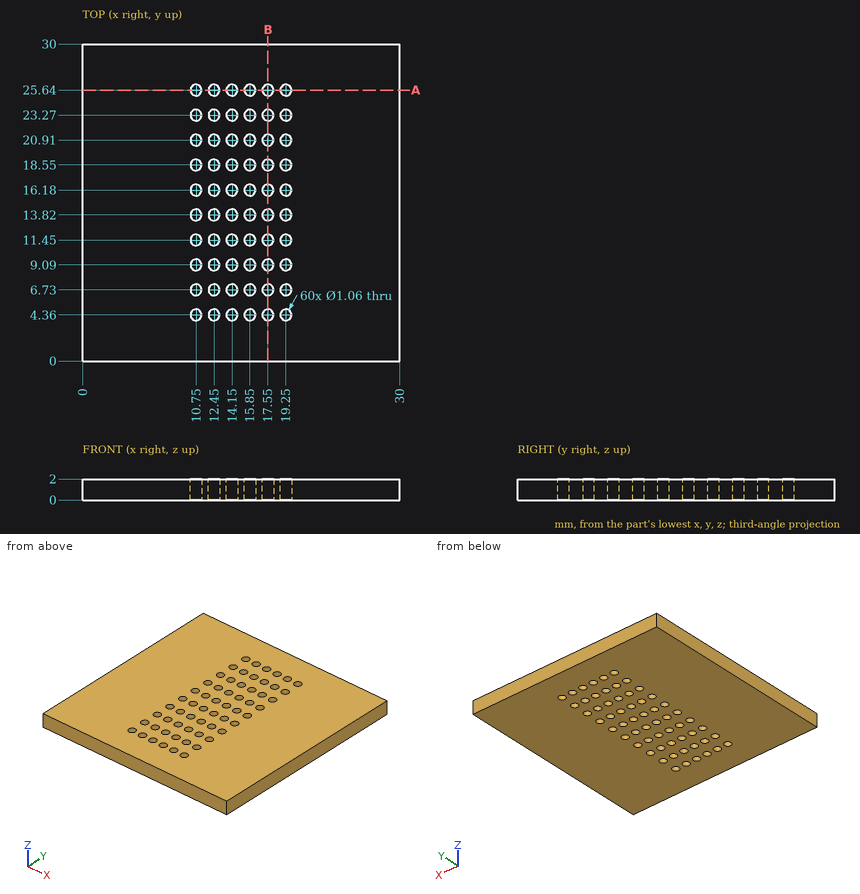
The drawing under review shows one solid part. Ordinate dimensions are in mm from its lowest x, y, z. Round coordinates to 2 decimals unless told otherwise and drop trailing zeros. Write each loop counter-clockwise with the first axis right and the second up, starting at its lowest first coordinate (ties: lowest second). Pieces come first, ordered by that corner, then holes. Notation, with made-up numbers: (1, 35) -> (22, 35) arc R8 cw to (22, 49) -> close; hole circle Ø9 at (31.5, 65.25). An arc over 180 degrees is marked (long way). One line per question, with ' | ' between items.
(1) Insertion check: P1, Ø1.2, axis at x = 12.45, y = 23.27, coming from the +Z side. The pin has a flat end and moves straight along its axis. Give the tip position at first contact, or say it passes through.
Result sheet:
P1: z = 2
(2) Take a section at B-B, the plane x = 17.55. State how many separate pieces and enclosed holes the cut face has, and give its area (3 significant figures).
Result sheet:
separate pieces: 11 | enclosed holes: 0 | area: 38.8 mm2
(3) Take a section at A-A, the plane y = 25.64. State the section outline as (x, z) points, and give its area (3 significant figures).
Result sheet:
outline: (0, 0) -> (10.22, 0) -> (10.22, 2) -> (0, 2) -> close; (11.28, 0) -> (11.92, 0) -> (11.92, 2) -> (11.28, 2) -> close; (12.98, 0) -> (13.62, 0) -> (13.62, 2) -> (12.98, 2) -> close; (14.68, 0) -> (15.32, 0) -> (15.32, 2) -> (14.68, 2) -> close; (16.38, 0) -> (17.02, 0) -> (17.02, 2) -> (16.38, 2) -> close; (18.08, 0) -> (18.72, 0) -> (18.72, 2) -> (18.08, 2) -> close; (19.78, 0) -> (30, 0) -> (30, 2) -> (19.78, 2) -> close | area: 47.3 mm2
